from build123d import *

# Parameters (mm, degrees)
F0_W      = 82.55
F0_H      = 38.1
F1_DEPTH  = 25.4
F2_W      = 28.575
F2_H      = 25.4
F3_DEPTH  = 25.4
F4_R      = 12.69999
F6_DEPTH  = 25.4
F8_DEPTH  = 25.4
F9_R      = 6.35
F10_DEPTH = 25.4
F11_R     = 6.35
F12_DEPTH = 25.4
F13_R     = 6.35
F14_DEPTH = 25.4


# Not quite as in the source:
# - a fillet or chamfer is up to 0.001 mm smaller than in the source, because OpenCascade refuses the exact size
# - a feature names something its author has since deleted; it is built from what else it names


with BuildPart() as f1:
    # F0 (on Front) → F1 (new body)
    with BuildSketch(Plane.XZ):
        with Locations((41.275, 19.05)):
            Rectangle(F0_W, F0_H)
    extrude(amount=F1_DEPTH)

    # F2 (on face) → F3 (cut)
    with BuildSketch(Plane.XZ.offset(25.4)):
        with Locations((14.2875, 25.4)):
            Rectangle(F2_W, F2_H)
        with Locations((68.2625, 25.4)):
            Rectangle(F2_W, F2_H)
    extrude(amount=-F3_DEPTH, mode=Mode.SUBTRACT)

    # F4 (radius 12.7 in the source; OpenCascade refuses exactly that, so slightly less here)
    f4_edges = [f1.edges().sort_by_distance(p)[0] for p in [
        (41.275, 0, 38.1),
        (41.275, -25.4, 38.1),
    ]]
    fillet(f4_edges, radius=F4_R)

    # F5 (on face) → F6 (cut)
    with BuildSketch(Plane.XY.offset(12.7)):
        with BuildLine():
            ThreePointArc((68.2625, 0), (77.4605547287, -12.7), (68.2625, -25.4))
            Line((68.2625, -25.4), (82.55, -25.4))
            Line((82.55, -25.4), (82.55, 0))
            Line((82.55, 0), (68.2625, 0))
        make_face()
    extrude(amount=-F6_DEPTH, mode=Mode.SUBTRACT)

    # F7 (on face) → F8 (cut)
    with BuildSketch(Plane.XY.offset(12.7)):
        with BuildLine():
            ThreePointArc((12.733777985, -25.4), (3.1920308375, -12.0688091081), (14.2875, 0))
            Line((14.2875, 0), (0, 0))
            Line((0, 0), (0, -25.4))
            Line((0, -25.4), (12.733777985, -25.4))
        make_face()
    extrude(amount=-F8_DEPTH, mode=Mode.SUBTRACT)

    # F9 (on face) → F10 (cut)
    with BuildSketch(Plane.XY.offset(12.7)):
        with Locations((66.675, -12.7)):
            Circle(F9_R)
    extrude(amount=-F10_DEPTH, mode=Mode.SUBTRACT)

    # F11 (on face) → F12 (cut)
    with BuildSketch(Plane.XY.offset(12.7)):
        with Locations((15.875, -12.7)):
            Circle(F11_R)
    extrude(amount=-F12_DEPTH, mode=Mode.SUBTRACT)

    # F13 (on face) → F14 (cut)
    with BuildSketch(Plane.YZ.offset(53.975)):
        with Locations((-12.7, 25.4)):
            Circle(F13_R)
    extrude(amount=-F14_DEPTH, mode=Mode.SUBTRACT)


solid = f1.part
The model under review builds one solid part; all positions refer to its coordinate system, in mm. A direction names the side the tool comes from. Round coordinates to 2 decimals unless told otherwise and drop trailing zeros. Write each loop counter-clockwise with the first axis right and the second up, starting at its lowest first coordinate (ties: lowest second). Pieces come first, ordered by that corner, then holes. Notation, with made-up numbers: M 74.5,-14.5 L 107.5,-14.5 A26 cw 107.5,12.5 Z; hole C 69.5,12 d4. An arc over 180 degrees is marked long. Answer as CSV lines item,"result". Start each with the question number.
Q1. Wall thickness on line 1 along Z through (x, y) = (45.25, -12.7); line 2 along X through (y, z) = (-10, 4.5); line 3 along Y through (x, z) = (37, 25): over which ranges is each line inside the solid? List them lowest first.
Q2. The part is to be moulded in two halves that separate along Y. For faces 4 (the face through (40, -25.4, 10)), 5 (the face through (60, -10, 12.7)), 6 (the face through (3.18, -12.32, 6.44)), 7 (the face through (18.81, -18.33, 6.44)), say which applies: +Y half, -Y half, draft (parallel to the pull), parting line (faces both ways), or undercut.
Q3. Tool access review of faces 1 (the face through (41.453, -9.77, 19.766)), 2 (the face through (53.975, -15.7, 19.6)), 3 (the face through (19, -19, 12.7)): name each direction out of +Z, -Z, +X, -X, +Y, -Y from which nothing blocks a thin tool from reaching the whole face with its end or side.
Q4. Consider section C-C, the plane y = -16.5. Give the boundary of the cut face in (x, z) (3 decimals), then the cut area to 3 significant figures.
Q5. Clearance check with flat-ended pins moving along their axes: P1, Ø1, axis at y = -3.5, z = 31.5, coming from the -X side (3 decimals); P2, Ø11.5, axis at x = 15.875, y = -12.7, coming from the -Z side; P3, Ø7.5, axis at x = 19, y = -12, coming from the +Z side; P4, Ø10, axis at y = -23, z = 30.5, coming from the +X side (3 decimals). State where each tip first meets the part, or that it passes through.
Q6. Consider section B-B, the plane x = 17. Give the boundary of the cut face in (y, z), then the cut area to 3 significant figures.
Q7. Consider section D-D, the plane y = -22.25. Give the boundary of the cut face in (x, z) (3 decimals), then the cut area to 3 significant figures.
Q8. Consider section A-A, the plane z = 30. Give the boundary of the cut face in (x, y) (1 decimal).
Result set:
1,line 1,"z = 0 to 19.05, 31.75 to 38.1"
1,line 2,"x = 3.49 to 10.13, 21.62 to 60.93, 72.42 to 77.19"
1,line 3,"y = -25.4 to -19.04, -6.36 to 0"
2,face 4,"-Y half"
2,face 5,"draft"
2,face 6,"parting line"
2,face 7,"undercut"
3,face 1,"+X, -X"
3,face 2,"+Z, +X, +Y, -Y"
3,face 3,"+Z, -X, +Y, -Y"
4,outline,"M 3.687,0 L 10.788,0 L 10.788,12.7 L 3.687,12.7 Z; M 20.962,0 L 61.588,0 L 61.588,12.7 L 53.975,12.7 L 53.975,20.313 L 28.575,20.313 L 28.575,12.7 L 20.962,12.7 Z; M 28.575,30.487 L 53.975,30.487 L 53.975,37.518 L 28.575,37.518 Z; M 71.762,0 L 76.909,0 L 76.909,12.7 L 71.762,12.7 Z"
4,area,"1,040 mm²"
5,P1,"stops at x = 28.575"
5,P2,"passes through"
5,P3,"stops at z = 12.7"
5,P4,"stops at x = 53.975"
6,outline,"M -25.4,0 L -18.95,0 L -18.95,12.7 L -25.4,12.7 Z; M -6.45,0 L 0,0 L 0,12.7 L -6.45,12.7 Z"
6,area,"164 mm²"
7,outline,"M 7.175,0 L 73.446,0 L 73.446,12.7 L 53.975,12.7 L 53.975,33.772 L 28.575,33.772 L 28.575,12.7 L 7.175,12.7 Z"
7,area,"1,380 mm²"
8,outline,"M 28.6,-24.5 L 54,-24.5 L 54,-17.1 L 28.6,-17.1 Z; M 28.6,-8.3 L 54,-8.3 L 54,-0.9 L 28.6,-0.9 Z"
